from build123d import *

# Parameters (mm, degrees)
SKETCH1_R           = 2.1
BOSS_EXTRUDE1_DEPTH = 215
FILLET1_R           = 2


with BuildPart() as part:
    # Sketch1 → Boss-Extrude1 (new body)
    with BuildSketch(Plane(origin=(0, 0, 0), x_dir=(0, 0, -1), z_dir=(1, 0, 0))):
        Polygon((87.447995492, 61.569861664), (99.124438977, 63.188614895), (97.476589763, 75.074934467), (86.155762657, 71.861000707), align=None)
        with Locations((93.379181481, 67.734629599)):
            Circle(SKETCH1_R, mode=Mode.SUBTRACT)
    extrude(amount=BOSS_EXTRUDE1_DEPTH)

    # Fillet1
    fillet1_edges = [part.edges().sort_by_distance(p)[0] for p in [
        (107.5, 63.188614895, -99.124438977),
    ]]
    fillet(fillet1_edges, radius=FILLET1_R)


solid = part.part
Here's how the part is built. I have some questions about the finished solid (model axes, mm). Coordinates: 2 decimals unless noted, no trailing zeros. Order: outer loops, then holes, each group sorted by start corner. A loop starts at its lowest first (then second) coordinate and runs counter-clockwise, first axis right, second up.
Item 1: If we mould it in two halves opening along Y, with no side actions, what happens to faces 1 (the face through (105.995, 69.505, -94.508)), 2 (the face through (0, 68, -91)), 3 (the face through (105.995, 66.787, -86.793))? For each: +Y half, -Y half, draft (parallel to the pull), parting line (faces both ways), or undercut.
Result sheet:
face 1: undercut
face 2: draft
face 3: -Y half
Item 2: If we section it at A-A on x = 87: List the corners of the cut face in (y, z) for me, plus the area to 3 significant figures.
Result sheet:
outline: (61.57, -87.45) - (62.91, -97.14) arc R2 ccw to (65.17, -98.85) - (75.07, -97.48) - (71.86, -86.16) - close; hole circle Ø4.2 at (67.73, -93.38)
area: 116 mm2
Item 3: I need wall thicknesses on line 1 (Y direction, x = 75.5, z = -92.25); line 2 (Z direction, x = 26.5, y = 69); line 3 (Y direction, x = 49.5, z = -95). Which ranges of each line are inside material? Lowest first, please.
Result sheet:
line 1: y = 62.24 to 65.96, 69.51 to 73.59
line 2: z = -98.32 to -95.06, -91.7 to -86.52
line 3: y = 62.62 to 66.4, 69.07 to 74.37
Item 4: For P1, Ø1.5, axis at x = 83, z = -87.5, coming from the -Y side; P2, Ø1, axis at x = 141.5, z = -94, coming from the +Y side; P3, Ø4, axis at x = 41.5, y = 70.5, coming from the -Z side; P4, Ø3, axis at x = 169.5, z = -96.5, coming from the -Y side, each with a flat end and sliding along its axis, tell me the tip position at first contact or that it passes through.
Result sheet:
P1: stops at y = 61.57
P2: stops at y = 74.23
P3: stops at z = -98.39
P4: stops at y = 62.62
